```python
from build123d import *

# Parameters (mm, degrees)
SKETCH1_R                                    = 31
BOSS_EXTRUDE1_DEPTH                          = 21.25
CUT_EXTRUDE1_DEPTH                           = 91
F_5_0MM_DOWEL_HOLE1_D                        = 5
F_5_0MM_DOWEL_HOLE1_DEPTH                    = 8
F_5_0MM_DOWEL_HOLE1_TIP                      = 1.502151548
CBORE_FOR_M8_HEX_HEAD_CAP_SCREW2_D           = 6.5
CBORE_FOR_M8_HEX_HEAD_CAP_SCREW2_CBORE_D     = 11
CBORE_FOR_M8_HEX_HEAD_CAP_SCREW2_CBORE_DEPTH = 13
SKETCH18_R                                   = 31
SKETCH18_R_2                                 = 27.58
BOSS_EXTRUDE2_DEPTH                          = 4
SKETCH21_R                                   = 3
CUT_EXTRUDE2_DEPTH                           = 122.617548954


with BuildPart() as part:
    # Sketch1 → Boss-Extrude1 (new, symmetric)
    with BuildSketch(Plane.XY):
        with BuildLine():
            Line((-99.665912553, 10.461014095), (-99.665912553, -6.377493087))
            Line((-99.665912553, -6.377493087), (-82.665912553, -6.377493087))
            Line((-82.665912553, -6.377493087), (-82.665912553, -66.377493087))
            Line((-82.665912553, -66.377493087), (11.670122046, -33.950231979))
            ThreePointArc((11.670122046, -33.950231979), (34.334087447, 10.487155916), (-9.291603719, 34.676737164))
            Line((-9.291603719, 34.676737164), (-99.665912553, 10.461014095))
        make_face()
        Circle(SKETCH1_R, mode=Mode.SUBTRACT)
    extrude(amount=BOSS_EXTRUDE1_DEPTH, both=True)

    # Sketch5 → Cut-Extrude1 (cut)
    with BuildSketch(Plane.ZY.offset(82.665912553)):
        Polygon((-21.25, -66.377493087), (8.75, -66.377493087), (-21.25, -36.377493087), align=None)
    extrude(amount=-CUT_EXTRUDE1_DEPTH, mode=Mode.SUBTRACT)

    # Ø5.0mm Dowel Hole1
    with Locations(Plane.ZY.offset(82.665912553)):
        with Locations((15.68, -60.677493087), (15.68, -36.677493087), (-98.628383383, 36.760601071), (0.68, -44.677493087), (35.6, -82.217865389)):
            Hole(F_5_0MM_DOWEL_HOLE1_D / 2, depth=F_5_0MM_DOWEL_HOLE1_DEPTH)
            with Locations((0, 0, -(F_5_0MM_DOWEL_HOLE1_DEPTH + F_5_0MM_DOWEL_HOLE1_TIP / 2))):  # 118° drill point
                Cone(0, F_5_0MM_DOWEL_HOLE1_D / 2, F_5_0MM_DOWEL_HOLE1_TIP, mode=Mode.SUBTRACT)

    # CBORE for M8 Hex Head Cap Screw2 (through all)
    with Locations(Plane(origin=(0, 17.622506913, 0), x_dir=(-1, 0, 0), z_dir=(0, 1, 0))):
        with Locations((87.965912553, -15.25), (87.965912553, 12.95)):
            CounterBoreHole(CBORE_FOR_M8_HEX_HEAD_CAP_SCREW2_D / 2, CBORE_FOR_M8_HEX_HEAD_CAP_SCREW2_CBORE_D / 2, CBORE_FOR_M8_HEX_HEAD_CAP_SCREW2_CBORE_DEPTH)

    # Sketch18 → Boss-Extrude2 (add, symmetric)
    with BuildSketch(Plane(origin=(0, 0, 0), x_dir=(-1, 0, 0), z_dir=(0, 0, -1))):
        Circle(SKETCH18_R)
        Circle(SKETCH18_R_2, mode=Mode.SUBTRACT)
    extrude(amount=BOSS_EXTRUDE2_DEPTH, both=True)

    # Sketch21 → Cut-Extrude2 (cut, through all)
    with BuildSketch(Plane(origin=(0, 0, 0), x_dir=(0, 0, -1), z_dir=(1, 0, 0))):
        with Locations(Location((0, 0, 0), (0, 0, 180))):
            Circle(SKETCH21_R)
    extrude(amount=CUT_EXTRUDE2_DEPTH, mode=Mode.SUBTRACT)


solid = part.part
```
Could you check a few things on this model? Use its own coordinates, in mm. A direction names the side the tool comes from. Round coordinates to 2 decimals unless told otherwise and drop trailing zeros. Loops run counter-clockwise (first coordinate to the right, second up) from the corner with the lowest first, then second, coordinate; pieces in that order, holes last.
Q1. Thinking about a two-plate mould opening in Z: for faces 1 (the flat face through (28, -2, 4)), 2 (the conical face through (-73.425, -36.247, 15.623)), 3 (the flat face through (-53.846, 22.738, 0.297)), which applies, pulls with the +Z half, pulls with the -Z half, needs draft (parallel to the pull), parting line crosses it, or undercut?
Q2. For P1, Ø7.5, axis at x = -87.97, z = -15.25, coming from the -Y side; P2, Ø12, axis at y = -11.5, z = 1.5, coming from the +X side; P3, Ø8.5, axis at x = -87.97, z = 12.95, coming from the +Y side, each with a flat end and sliding along its axis, tell me the tip position at first contact or that it passes through.
Q3. I want a section at C-C (z = -15.25). Write out the boundary of the cut face in (x, y).
Q4. I want a section at A-A (y = 0). Write out the boundary of the cut face in (x, z), and give its area (3 significant figures).
Q5. On a 3-axis mill with a long thin cutter (end or side, diameter ignored), from which of +Z, -Z, +X, -X, +Y, -Y can I reach the whole of each face in a straight line? I mean faces 4 (the cylindrical face through (-78.61, -47.12, 1.22)), 5 (the cylindrical face through (-82.47, 8.81, 13.19)), 6 (the flat face through (28, -2, -4)). Say none if no direction works.
Q6. I want a section at B-B (x = 0). Write out the boundary of the cut face in (y, z), and give its area (3 significant figures).
Q7. I want a section at D-D (x = 19). Write out the boundary of the cut face in (y, z), and give its area (3 significant figures).
Q8. Please list where these lines run through material, in increasing order: L1, parallel to X at y = -5, z = 14; L2, parallel to X at y = -10.5, z = 7; L3, parallel to Y at x = -7.5, z = -14.
Answer below:
1. face 1: pulls with the +Z half
1. face 2: undercut
1. face 3: needs draft
2. P1: stops at y = -6.38
2. P2: stops at x = 35.48
2. P3: stops at y = 4.62
3. outline: (-99.67, -6.38) - (-91.22, -6.38) - (-91.22, 4.62) - (-93.47, 4.62) - (-93.47, 12.12) - (-99.67, 10.46) - close; (-84.72, -6.38) - (-82.67, -6.38) - (-82.67, -42.38) - (-12.85, -42.38) - (11.67, -33.95) arc R35.9 ccw to (-9.29, 34.68) - (-82.47, 15.07) - (-82.47, 4.62) - (-84.72, 4.62) - close; hole circle Ø62 at (0, 0)
4. outline: (-99.67, -21.25) - (-31, -21.25) - (-31, -4) - (-27.58, -4) - (-27.58, 4) - (-31, 4) - (-31, 21.25) - (-99.67, 21.25) - close; (27.58, -4) - (31, -4) - (31, -21.25) - (35.9, -21.25) - (35.9, -3) - (27.58, -3) - close; (27.58, 3) - (35.9, 3) - (35.9, 21.25) - (31, 21.25) - (31, 4) - (27.58, 4) - close; hole circle Ø6.5 at (-87.97, -15.25); hole circle Ø6.5 at (-87.97, 12.95)
4. area: 3,060 mm2
5. face 4: -X
5. face 5: +Y
5. face 6: -Z
6. outline: (-37.96, -19.67) - (-36.38, -21.25) - (-31, -21.25) - (-31, -4) - (-27.58, -4) - (-27.58, 4) - (-31, 4) - (-31, 21.25) - (-37.96, 21.25) - close; (27.58, -4) - (31, -4) - (31, -21.25) - (35.9, -21.25) - (35.9, 21.25) - (31, 21.25) - (31, 4) - (27.58, 4) - close
6. area: 558 mm2
7. outline: (-30.46, -21.25) - (-24.49, -21.25) - (-24.49, -4) - (-19.99, -4) - (-19.99, 4) - (-24.49, 4) - (-24.49, 21.25) - (-30.46, 21.25) - close; (19.99, -4) - (24.49, -4) - (24.49, -21.25) - (30.46, -21.25) - (30.46, 21.25) - (24.49, 21.25) - (24.49, 4) - (19.99, 4) - close
7. area: 579 mm2
8. L1: x = -99.67 to -91.04, -84.89 to -30.59, 30.59 to 35.55
8. L2: x = -82.67 to -29.17, 29.17 to 34.33
8. L3: y = -40.54 to -30.08, 30.08 to 35.11
